Autodesk Fusion 360 part; units mm, degrees
sketch "Sketch2" plane through (5, 0, 0) normal (1, 0, 0) x (0, 1, 0)
  line L0 (16.9637, 18.2844) -> (-13.0292, -11.7227) construction
  line L1 (-12.9363, 18.2856) -> (17.0619, -11.7162) construction
  circle A0 centre (13.0169, 14.3306) radius 1.6
  circle A1 centre (-8.9831, 14.3306) radius 1.6
  circle A2 centre (-8.9831, -7.6694) radius 1.6
  circle A3 centre (13.0169, -7.6694) radius 1.6
  circle A4 centre (-8.9831, 14.3306) radius 4.1
  circle A5 centre (13.0169, 14.3306) radius 4.1
  circle A6 centre (-8.9831, -7.6694) radius 4.1
  line L2 (9.4619, 10.7862) -> (-5.5274, -4.2245) construction
  line L3 (-6.6835, 17.7249) -> (2.0169, 11.8306)
  line L4 (2.0169, 11.8306) -> (10.7173, 17.7249)
  line L5 (-12.3753, 12.0277) -> (-6.471, 3.3306)
  line L6 (-6.471, 3.3306) -> (-12.3753, -5.3666)
  line L7 (-6.6835, -11.0638) -> (2.0169, -5.1694)
  line L8 (10.5048, 3.3306) -> (16.4091, 12.0277)
  circle A7 centre (13.0169, -7.6694) radius 4.1
  line L9 (10.5048, 3.3306) -> (16.4091, -5.3666)
  line L10 (2.0169, -5.1694) -> (10.7173, -11.0638)
  line L11 (-4.4831, -3.1694) -> (8.5169, -3.1694)
  line L12 (8.5169, -3.1694) -> (8.5169, 9.8306)
  line L13 (8.5169, 9.8306) -> (-4.4831, 9.8306)
  line L14 (-4.4831, 9.8306) -> (-4.4831, -3.1694)
  line L15 (-4.4831, -3.1694) -> (8.5169, 9.8306) construction
  line L16 (8.5169, -3.1694) -> (-4.4831, 9.8306) construction
  line L17 (10.5048, 11.8306) -> (-6.471, 11.8306)
  line L18 (-6.471, 11.8306) -> (-6.471, -5.1694)
  line L19 (-6.471, -5.1694) -> (10.5048, -5.1694)
  line L20 (10.5048, -5.1694) -> (10.5048, 11.8306)
  line L21 (10.5048, 11.8306) -> (-6.471, -5.1694) construction
  line L22 (-6.471, 11.8306) -> (10.5048, -5.1694) construction
  point P0 (2.0169, 3.3306)
  point P1 (2.0169, 3.3306)
  point P2 (2.0169, 3.3306)
  point P3 (2.0169, 3.3306)
  point P4 (2.0169, 3.3306)
  dimension "d11" = 3.2
  dimension "d12" = 11
  dimension "d13" = 3.2
  dimension "d14" = 3.2
  dimension "d15" = 3.2
  dimension "d18" = 11
  dimension "d19" = 22
  dimension "d20" = 8.2
  dimension "d21" = 8.2
  dimension "d22" = 8.2
  dimension "d23" = 8.2
  dimension "d33" = 13
  dimension "d34" = 17
  dimension "d35" = 22
extrude "Extrude8" add sketch "Sketch2" along normal blind 5 contours A4 L17 L18 | A4 L3 L17 | A4 A5 A6 A7 L17 L18 L19 L20 | A4 L17 L18 | A4 L5 L18 | A5 L4 L17 | A6 L6 L18 | A5 L17 L20 | A5 L17 L20 | A6 L18 L19 | A6 L18 L19 | A5 L8 L20 | A6 L7 L19 | A7 L9 L20 | A7 L10 L19 | A7 L19 L20 | A7 L19 L20 | L11 L12 L13 L14
extrude "Extrude9" add sketch "Sketch2" against normal blind 5 contours A4 A5 A6 A7 L17 L18 L19 L20
extrude "Extrude10" cut sketch "Sketch2" along normal blind 5 contours L11 L12 L13 L14
extrude "Extrude3" [suppressed]
equation "d11 = motorScrewHole"
equation "d12 = ( 22 / 2 ) * 1 mm"
equation "d13 = motorScrewHole"
equation "d14 = motorScrewHole"
equation "d15 = motorScrewHole"
equation "motorScrewHole = 3.2 mm"
equation "d18 = ( 22 / 2 ) * 1 mm"
equation "d20 = motorScrewHole + 5 mm"
equation "d21 = motorScrewHole + 5 mm"
equation "d22 = motorScrewHole + 5 mm"
equation "d23 = motorScrewHole + 5 mm"
Here's how the part is built. I have some questions about the finished solid (model axes, mm). A direction names the side the tool comes from. Give positions to 0.01 mm unless a question says otherwise; leave off trailing zeros. Loops run counter-clockwise (first coordinate to the right, second up) from the corner with the lowest first, then second, coordinate; pieces in that order, holes last. Notation, with made-up numbers: M 6,71.5 L 51,71.5 A22 cw 51,102.5 Z; hole C -24.75,30 d4. An arc over 180 degrees is marked long. Put each result on its own line as item: value. Start each with the question number.
(1) If we mould it in two halves opening along Z, with no side actions, what happens to faces 5 (the flat face through (5, 11, -6)), 6 (the flat face through (7.46, 6.31, 14.74)), 7 (the flat face through (7.465, 13.416, -0.957))? For each: +Z half, -Z half, draft (parallel to the pull), parting line (faces both ways), or undercut.
(2) I need wall thicknesses on line 1 along Z through (x, y) = (7, 13.5); line 2 along Z through (x, y) = (3, -3); line 3 along Y through (x, z) = (1.5, 3.5). Which ranges of each line are inside material? Lowest first, please. Write a range as [from, to].
(3) I want a section at D-D on z = 4.5. Please give me the cut outline in (x, y).
(4) I want a section at A-A on x = 2.75. Please give me the cut outline in (y, z), then the cut area to 3 significant figures.
(5) I want a section at C-C on z = -7. Please give me the cut outline in (x, y).
(6) Will these pins go through, and if not, where does the flat tip stop? pin 1 Ø4 at (x, y) = (2.5, 1) entering from -Z; pin 2 Ø3.5 at (y, z) = (-8.98, -7.67) entering from -X; pin 3 Ø1 at (x, z) = (7.5, 6.5) entering from +Y; pin 4 Ø2.5 at (y, z) = (-8.98, 14.33) entering from +X.
(7) I want a section at B-B on y = 1. Please give me the cut outline in (x, z).
(8) For faces 1 (the flat face through (7.465, 13.416, 7.618)), 2 (the flat face through (3, 2, -5.169)), 3 (the flat face through (3, 10.505, 3)), 4 (the flat face through (5, -7, -6)), which set-ups out of +Z, -Z, +X, -X, +Y, -Y let a thin tool reach every point of the face, with its end or its side?
Answer block:
1. face 5: draft
1. face 6: +Z half
1. face 7: undercut
2. line 1: [-11.74, -9.19], [-6.14, -1.08], [7.74, 12.81], [15.86, 18.4]
2. line 2: [-5.17, -3.17], [9.83, 11.83]
2. line 3: [-6.47, -4.48], [8.52, 10.5]
3. outline: M 0,-6.47 L 5,-6.47 L 5,-7.26 L 10,-7.26 L 10,-4.48 L 0,-4.48 Z; M 0,8.52 L 10,8.52 L 10,11.3 L 5,11.3 L 5,10.5 L 0,10.5 Z
4. outline: M -6.47,-4.43 A4.1 cw -5.73,-5.17 L 9.77,-5.17 A4.1 cw 10.5,-4.43 L 10.5,11.09 A4.1 cw 9.77,11.83 L -5.73,11.83 A4.1 cw -6.47,11.09 Z; hole M -4.48,-3.17 L 8.52,-3.17 L 8.52,9.83 L -4.48,9.83 Z
4. area: 118 mm^2
5. outline: M 5,-13.03 L 10,-13.03 L 10,-10.44 L 5,-10.44 Z; M 5,-7.53 L 10,-7.53 L 10,-0.69 L 5,-0.69 Z; M 5,4.72 L 10,4.72 L 10,11.56 L 5,11.56 Z; M 5,14.47 L 10,14.47 L 10,17.06 L 5,17.06 Z
6. pin 1: z = -5.17
6. pin 2: x = 5
6. pin 3: y = 13
6. pin 4: through
7. outline: M 0,-5.17 L 5,-5.17 L 5,-5.86 L 10,-5.86 L 10,-3.17 L 0,-3.17 Z; M 0,9.83 L 10,9.83 L 10,12.52 L 5,12.52 L 5,11.83 L 0,11.83 Z
8. face 1: +X, -X, +Y
8. face 2: -Z, -X, +Y, -Y
8. face 3: +Z, -Z, -X, +Y
8. face 4: -Z, -X, -Y
